Work out the finished part from the listing and answer in its coordinate system (mm). A direction names the side the tool comes from. Give positions to 0.01 mm unless a question says otherwise; leave off trailing zeros. Write each loop counter-clockwise with the first axis right and the second up, starting at its lowest first coordinate (ties: lowest second). Pieces come first, ordered by that corner, then holes.
1) Straight lines are drawn through the part: probe 1 along Y at (x, z) = (30.5, 1.55); probe 2 along Y at (x, z) = (31, 1.7); probe 3 along Y at (x, z) = (39, 2.3). For each, find the intervals that lie inside material, in ascending order.
2) Find section B-B (x = 31). Determine the outline of the cut face in (y, z), plus the area to 3 significant figures.
3) Determine the mould class of faces 1 (the face through (10, 38.212, 1)), 2 (the face through (31.886, 27.265, 1.479)), 3 (the face through (4.453, 41.642, 1.479)) for opening direction Y: pulls with the +Y half, pulls with the -Y half, needs draft (parallel to the pull), parting line crosses it, or undercut.
4) Find section D-D (z = 1.7). Determine the outline of the cut face in (x, y), plus the area to 3 significant figures.
5) Find section C-C (y = 52). Determine the outline of the cut face in (x, z).
6) Given pin 1 Ø0.9 at (x, z) = (10.5, 1.5) entering from -Y; pin 2 Ø1.5 at (y, z) = (16.5, 2) entering from -X, each flat-ended and moving along its own axis, determine where each tip first touches the part or whether it passes through.
7) A tool of negligible diameter and unlimited length cuts with its end or side. For faces 4 (the face through (51, 43.3, 1.5)), 5 (the face through (30.046, 8.064, 0.493)), 6 (the face through (50, 38.212, 1)), from which of +Z, -Z, +X, -X, +Y, -Y can it reach the whole face along a straight path? Write none if from no direction.
8) Find section A-A (x = 41). Determine the outline of the cut face in (y, z), plus the area to 3 significant figures.
```python
from build123d import *

# Parameters (mm, degrees)
CORTE_EXTERIOR_R        = 3.500002593
SALIENTE_EXTRUIR1_DEPTH = 3
CORTAR_EXTRUIR1_DEPTH   = 1
CORTAR_EXTRUIR2_DEPTH   = 0.1


with BuildPart() as part:
    # Corte exterior → Saliente-Extruir1 (new body)
    with BuildSketch(Plane.XY):
        with BuildLine():
            Line((47.504320945, 38.211786495), (51.847305041, 38.211786495))
            ThreePointArc((51.847305041, 38.211786495), (55.534254627, 41.572373104), (54.480090972, 46.448424641))
            ThreePointArc((54.480090972, 46.448424641), (30.004320476, 57.31391234), (5.528550918, 46.448424641))
            ThreePointArc((5.528550918, 46.448424641), (4.474387263, 41.572373104), (8.161336848, 38.211786495))
            Line((8.161336848, 38.211786495), (12.511035037, 38.211786495))
            ThreePointArc((12.511035037, 38.211786495), (15.339462162, 37.04021362), (16.511035037, 34.211786495))
            Line((16.511035037, 34.211786495), (16.504320945, -26.686088981))
            ThreePointArc((16.504320945, -26.686088981), (17.67589382, -29.514516106), (20.504320945, -30.686088981))
            Line((20.504320945, -30.686088981), (39.504320945, -30.686088981))
            ThreePointArc((39.504320945, -30.686088981), (42.33274807, -29.514516106), (43.504320945, -26.686088981))
            Line((43.504320945, -26.686088981), (43.504320945, 34.211786495))
            ThreePointArc((43.504320945, 34.211786495), (44.67589382, 37.04021362), (47.504320945, 38.211786495))
        make_face()
        with Locations((30.00431952, 24.313911283)):
            Circle(CORTE_EXTERIOR_R, mode=Mode.SUBTRACT)
        with BuildLine():
            ThreePointArc((52.277272453, 44.456319148), (30.004320476, 54.343913397), (7.731367869, 44.456320565))
            Line((7.731367869, 44.456320565), (10.253113799, 42.175794866))
            ThreePointArc((10.253113799, 42.175794866), (30.004320476, 50.943913397), (49.755526523, 42.175793449))
            Line((49.755526523, 42.175793449), (52.277272453, 44.456319148))
        make_face(mode=Mode.SUBTRACT)
    extrude(amount=SALIENTE_EXTRUIR1_DEPTH)

    # Grabado Superficie → Cortar-Extruir1 (cut)
    with BuildSketch(Plane.XY):
        with BuildLine():
            Line((32.873672963, 22.309708905), (31.999357171, 9.92309063))
            ThreePointArc((31.999357171, 9.92309063), (30.004320945, 8.063911283), (28.009284719, 9.92309063))
            Line((28.009284719, 9.92309063), (27.134968927, 22.309708905))
            ThreePointArc((27.134968927, 22.309708905), (30.004320945, 20.813910115), (32.873672963, 22.309708905))
        make_face()
    extrude(amount=CORTAR_EXTRUIR1_DEPTH, mode=Mode.SUBTRACT)

    # grabado linea medio → Cortar-Extruir2 (cut)
    with BuildSketch(Plane.XY):
        Polygon((43.479990352, -26.052604982), (35.339991301, -26.048672531), (35.337749708, -30.68867199), (32.817750002, -30.687454573), (32.819992183, -26.046238615), (16.48009071, -25.838344751), (16.491215962, -2.809563938), (32.831214056, -2.817457825), (32.833455649, 1.822541634), (35.353455355, 1.821324216), (35.351213761, -2.818675242), (39.411213288, -2.820636636), (39.407309823, -10.900635693), (43.487309347, -10.90260675), align=None)
    extrude(amount=CORTAR_EXTRUIR2_DEPTH, mode=Mode.SUBTRACT)


solid = part.part
```
Results:
1. probe 1: y = -30.69 to 20.85, 27.78 to 50.94, 54.34 to 57.31
1. probe 2: y = -30.69 to 20.96, 27.67 to 50.93, 54.33 to 57.3
1. probe 3: y = -30.69 to 49.38, 52.96 to 56.06
2. outline: (-30.69, 0) - (-26.02, 0) - (-26.02, 0.1) - (-2.82, 0.1) - (-2.82, 0) - (8.33, 0) - (8.33, 1) - (20.96, 1) - (20.96, 3) - (-30.69, 3) - close; (27.67, 0) - (50.93, 0) - (50.93, 3) - (27.67, 3) - close; (54.33, 0) - (57.3, 0) - (57.3, 3) - (54.33, 3) - close
2. area: 219 mm2
3. face 1: pulls with the -Y half
3. face 2: undercut
3. face 3: parting line crosses it
4. outline: (5.53, 46.45) arc R5 ccw to (8.16, 38.21) - (12.51, 38.21) arc R4 cw to (16.51, 34.21) - (16.5, -26.69) arc R4 ccw to (20.5, -30.69) - (39.5, -30.69) arc R4 ccw to (43.5, -26.69) - (43.5, 34.21) arc R4 cw to (47.5, 38.21) - (51.85, 38.21) arc R5 ccw to (54.48, 46.45) arc R33 ccw to start; hole (7.73, 44.46) - (10.25, 42.18) arc R26.63 cw to (49.76, 42.18) - (52.28, 44.46) arc R30.03 ccw to start; hole circle Ø7 at (30, 24.31)
4. area: 2,440 mm2
5. outline: (12.05, 0) - (18.37, 0) - (18.37, 3) - (12.05, 3) - close; (41.64, 0) - (47.96, 0) - (47.96, 3) - (41.64, 3) - close
6. pin 1: stops at y = 38.21
6. pin 2: stops at x = 16.51
7. face 4: +Z, -Z
7. face 5: -Z
7. face 6: +Z, -Z, +X, -Y
8. outline: (-30.4, 0) - (-26.05, 0) - (-26.05, 0.1) - (-10.9, 0.1) - (-10.9, 0) - (48.57, 0) - (48.57, 3) - (-30.4, 3) - close; (52.26, 0) - (55.43, 0) - (55.43, 3) - (52.26, 3) - close
8. area: 245 mm2
